Verification items for the finished model (mm, model axes). A direction names the side the tool comes from. Round coordinates to 2 decimals unless told otherwise and drop trailing zeros. Order: outer loops, then holes, each group sorted by start corner. A loop starts at its lowest first (then second) coordinate and runs counter-clockwise, first axis right, second up. Notation, with made-up numbers: (73.25, 10) -> (87.25, 10) arc R21 ccw to (87.25, 22) -> close; hole circle Ø5 at (65, 47). An arc over 180 degrees is marked (long way). Return JSON: item names as keys, results as strings. Group by question number.
1) Tool access check on faces 1 (the flat face through (-6, 3, -0.461)), 2 (the flat face through (-10.84, 1.36, -12.31)), 3 (the flat face through (-8.795, 2.822, -6.964)), 4 (the flat face through (-8.6, 4.85, -5.7)), 5 (the flat face through (-10.84, 4.34, -12.31)). Record the directions out of +Z, -Z, +X, -X, +Y, -Y that give a thin tool (end or side, any length) a straight path to the whole face; none if there is none.
2) Section check A-A on x = 1.5. Enter the section's corners in (y, z).
3) Section check C-C on z = -4.5. Enter the section's corners in (x, y), plus the area to 3 significant figures.
4) Section check B-B on y = 2.9. State how many separate pieces and enclosed holes the cut face has, plus the area to 3 significant figures.
5) Draft check along Z on faces 6 (the cylindrical face through (-0.917, 2.89, -8.674)), 7 (the flat face through (-9.18, 2.82, -6.54)), 8 (the flat face through (-3, 0, -6)). Enter one of: pulls with the +Z half, pulls with the -Z half, needs draft (parallel to the pull), parting line crosses it, or undercut.
6) Depth check by flat-ended pin: pin 1 (0.5 mm diameter, centred on x = 2, z = -6.5, fed in from +Y); pin 2 (0.5 mm diameter, centred on x = 1, z = -1.5, fed in from -Y); pin 3 (0.5 mm diameter, centred on x = 2, y = 3, fed in from +Z). Enter the tip coordinate at first touch or a pass-through.
7) Scan lines: L1, parallel to Z at x = -0.7, y = 2.3; L2, parallel to X at y = 1.35, z = -9.65; L3, parallel to X at y = 3.9, z = -3.15. Record each from-to range of solid material in increasing order.
8) Section check D-D on z = -9.65. Enter the section's corners in (x, y), plus the area to 3 significant figures.
Autodesk Inventor part; units mm, degrees
ref_plane "Work Plane1" through (0, 2.85, 0) normal (0, 1, 0) x (1, 0, 0)
ref_plane "YZ Plane" through (0, 0, 0) normal (1, 0, 0) x (0, 1, 0)
ref_plane "XZ Plane" through (0, 0, 0) normal (0, 1, 0) x (-1, 0, 0)
sketch "Sketch1" plane through (0, 0, 0) normal (0, 1, 0) x (-1, 0, 0)
  line L0 (0, 0) -> (5.8, 0)
  line L1 (5.8, 0) -> (5.8, -12.8)
  line L2 (5.8, -12.8) -> (0, -12.8)
  line L3 (0, -12.8) -> (0, 0)
  dimension "d0" = 5.8
  dimension "d1" = 12.8
extrude "Extrusion1" add sketch "Sketch1" along normal blind 5.7
sketch "Sketch2" plane through (0, 5.7, 0) normal (0, 1, 0) x (1, 0, 0)
  circle A0 centre (-1.4, 3.15) radius 1
  line L0 (-5.8, 12.8) -> (-5.8, 0)
  line L1 (-5.8, 6.4) -> (0, 6.4) construction
  line L2 (0, 0) -> (0, 12.8)
  circle A1 centre (-1.4, 9.65) radius 1
  dimension "d4" = 2
  dimension "d5" = 3.25
  dimension "d6" = 1.4
extrude "Extrusion2" [suppressed]
sketch "Sketch3" plane through (0, 5.7, 0) normal (0, 1, 0) x (1, 0, 0)
  line L0 (0, 0) -> (0, 12.8)
  line L1 (0, 2.15) -> (0.7, 2.15)
  line L2 (0.7, 2.15) -> (0.7, 4.15)
  line L3 (0.7, 4.15) -> (0, 4.15)
  line L4 (0, 4.15) -> (0, 2.15)
  line L5 (0, 6.4) -> (-5.8, 6.4) construction
  line L6 (-5.8, 12.8) -> (-5.8, 0)
  circle A0 centre (-1.4, 3.15) radius 1
  line L7 (-1.4, 3.15) -> (-5.8, 3.15) construction
  line L8 (0.7, 3.15) -> (0, 3.15) construction
  line L9 (0, 10.65) -> (0.7, 10.65)
  line L10 (0.7, 10.65) -> (0.7, 8.65)
  line L11 (0.7, 8.65) -> (0, 8.65)
  line L12 (0, 8.65) -> (0, 10.65)
  line L13 (0.7, 9.65) -> (0, 9.65) construction
  point P0 (0, 8.65)
  point P1 (0, 4.15)
  dimension "d9" = 0.7
  dimension "d10" = 2
extrude "Extrusion3" add sketch "Sketch3" against normal blind 5.7 contours L0 L9 L10 L11 | L0 L3 L2 L1
chamfer "Chamfer1" distance 0.7 angle 45 4 edges at (0, 2.85, -4.15) (0, 2.85, -10.65) (0, 2.85, -8.65) (0, 2.85, -2.15)
sketch "Sketch4" plane through (0, 5.7, 0) normal (0, 1, 0) x (1, 0, 0)
  line L0 (0.7, 4.15) -> (0.7, 2.15)
  line L1 (0.7, 3.15) -> (-0.7, 3.15) construction
  circle A0 centre (-0.7, 3.15) radius 1
  line L2 (0, 4.85) -> (0, 7.95)
  line L3 (0, 6.4) -> (-5.8, 6.4) construction
  line L4 (-5.8, 12.8) -> (-5.8, 0)
  circle A1 centre (-0.7, 9.65) radius 1
  point P0 (0, 0)
  dimension "d16" = 2
  dimension "d17" = 1.4
extrude "Extrusion4" cut sketch "Sketch4" against normal blind 5.7
sketch "Sketch7" plane through (0, 0, -4.85) normal (1, 0, 0) x (0, 0, -1)
  line L0 (7.95, 5.7) -> (-4.85, 5.7)
  line L1 (1.55, 5.7) -> (1.55, 0) construction
  line L2 (1.25, 2.55) -> (1.85, 2.55)
  line L3 (1.85, 2.55) -> (1.85, 3.15)
  line L4 (1.85, 3.15) -> (1.25, 3.15)
  line L5 (1.25, 3.15) -> (1.25, 2.55)
  line L6 (1.25, 2.55) -> (1.85, 3.15) construction
  line L7 (1.85, 2.55) -> (1.25, 3.15) construction
  point P0 (-4.85, 0)
  point P1 (1.55, 2.85)
  dimension "d24" = 0.6
  dimension "d25" = 0.6
extrude "Extrusion6" add sketch "Sketch7" along normal blind 3.5
pattern_linear "Rectangular Pattern1" count 2 spacing 5 along (0, 0, -1) count 2 spacing 5 along (0, 0, 1) of "Extrusion6"
ref_plane "Work Plane1" through (0, 2.85, 0) normal (0, 1, 0) x (1, 0, 0)
sketch "Sketch8" plane through (0, 2.85, 0) normal (0, 1, 0) x (1, 0, 0)
  line L0 (-5.8, 12.8) -> (-5.8, 0)
  line L1 (-5.8, 0.4613) -> (-7.1649, 0.4613)
  line L2 (-7.1649, 0.4613) -> (-11.2583, 12.8)
  line L3 (-11.2583, 12.8) -> (-10.7315, 12.8)
  line L4 (-10.7315, 12.8) -> (-6.804, 0.9613)
  line L5 (-6.804, 0.9613) -> (-5.8, 0.9613)
  line L6 (0, 12.8) -> (-5.8, 12.8)
  point P0 (0, 0)
  dimension "d36" = 0.5
  dimension "d37" = 0.5
  dimension "d38" = 13
extrude "Extrusion7" add sketch "Sketch8" along normal mid plane 4
chamfer "Chamfer2" distance 1 angle 45 2 edges at (-10.9949, 4.85, -12.8) (-10.9949, 0.85, -12.8)
properties part number "Microswitch"
Check result:
{
 "1": {"face 1": "+Z, -X, +Y, -Y", "face 2": "-Z, -X, -Y", "face 3": "-Z, +Y, -Y", "face 4": "+Z, -Z, -X, +Y", "face 5": "-Z, -X, +Y"},
 "2": {"outline": "(2.55, -11.7) -> (3.15, -11.7) -> (3.15, -11.1) -> (2.55, -11.1) -> close; (2.55, -6.7) -> (3.15, -6.7) -> (3.15, -6.1) -> (2.55, -6.1) -> close; (2.55, -1.7) -> (3.15, -1.7) -> (3.15, -1.1) -> (2.55, -1.1) -> close"},
 "3": {"outline": "(-8.5, 0.85) -> (-7.98, 0.85) -> (-7.98, 4.85) -> (-8.5, 4.85) -> close; (-5.8, 0) -> (0.35, 0) -> (0.35, 5.7) -> (-5.8, 5.7) -> close", "area": "37.2 mm^2"},
 "4": {"separate pieces": "1", "enclosed holes": "2", "area": "84.9 mm^2"},
 "5": {"face 6": "undercut", "face 7": "pulls with the +Z half", "face 8": "needs draft"},
 "6": {"pin 1": "y = 3.15", "pin 2": "y = 2.55", "pin 3": "z = -1.1"},
 "7": {"L1": "-12.8 to -10.65, -8.65 to -4.15, -2.15 to 0", "L2": "-10.21 to -9.69, -5.8 to -1.7, 0.3 to 0.7", "L3": "-8.06 to -7.53, -5.8 to -1.7, 0.3 to 0.7"},
 "8": {"outline": "(-10.21, 0.85) -> (-9.69, 0.85) -> (-9.69, 4.85) -> (-10.21, 4.85) -> close; (-5.8, 0) -> (-1.7, 0) -> (-1.7, 5.7) -> (-5.8, 5.7) -> close; (0.3, 0) -> (0.7, 0) -> (0.7, 5.7) -> (0.3, 5.7) -> close", "area": "27.8 mm^2"}
}
